from build123d import *

# Parameters (mm, degrees)
SKETCH1_R           = 5
SKETCH1_R_2         = 4.5
BOSS_EXTRUDE1_DEPTH = 15
SKETCH2_R           = 10.85
BOSS_EXTRUDE2_DEPTH = 3.5
SKETCH4_R           = 1.75
CUT_EXTRUDE1_DEPTH  = 15.5
SKETCH5_R           = 4.5
CUT_EXTRUDE2_DEPTH  = 15.5


with BuildPart() as part:
    # Sketch1 → Boss-Extrude1 (new body)
    with BuildSketch(Plane.XY):
        Circle(SKETCH1_R)
        Circle(SKETCH1_R_2, mode=Mode.SUBTRACT)
    extrude(amount=BOSS_EXTRUDE1_DEPTH)

    # Sketch2 → Boss-Extrude2 (add)
    with BuildSketch(Plane.XY.offset(4.5)):
        Circle(SKETCH2_R)
    extrude(amount=-BOSS_EXTRUDE2_DEPTH)

    # Sketch4 → Cut-Extrude1 (cut)
    with BuildSketch(Plane.XY.offset(4.5)):
        with Locations((0, 7.6)):
            Circle(SKETCH4_R)
        with Locations((7.6, 0)):
            Circle(SKETCH4_R)
        with Locations((0, -7.6)):
            Circle(SKETCH4_R)
        with Locations((-7.6, 0)):
            Circle(SKETCH4_R)
    extrude(amount=-CUT_EXTRUDE1_DEPTH, mode=Mode.SUBTRACT)

    # Sketch5 → Cut-Extrude2 (cut)
    with BuildSketch(Plane(origin=(0, 0, 1), x_dir=(-1, 0, 0), z_dir=(0, 0, -1))):
        with Locations(Location((0, 0, 0), (0, 0, 180))):
            Circle(SKETCH5_R)
    extrude(amount=-CUT_EXTRUDE2_DEPTH, mode=Mode.SUBTRACT)


solid = part.part
The model under review builds one solid part; all positions refer to its coordinate system, in mm. A direction names the side the tool comes from. Give positions to 0.01 mm unless a question says otherwise; leave off trailing zeros. Order: outer loops, then holes, each group sorted by start corner. A loop starts at its lowest first (then second) coordinate and runs counter-clockwise, first axis right, second up. Notation, with made-up numbers: M -40,58.25 L 8,58.25 A11 ccw 8,69.25 Z; hole C 2.25,12.5 d7. An arc over 180 degrees is marked long. One line per question, with ' | ' between items. Start each with the question number.
1) Wall thickness on L1, parallel to X at y = 0.25, z = 9.5; L2, parallel to X at y = -1.5, z = 4.25; L3, parallel to Y at x = 0, z = 12: over which ranges is each line inside the solid? List them lowest first. Write a range as from..to.
2) Clearance check with flat-ended pins moving along their axes: P1, Ø2, axis at x = -7.6, y = 0, coming from the -Z side; P2, Ø4, axis at x = 7.6, y = 0, coming from the +Z side; P3, Ø2, axis at y = -3, z = 12, coming from the +X side; P4, Ø4, axis at y = -5, z = 2, coming from the -X side. State where each tip first meets the part, or that it passes through.
3) Consider section C-C, the plane y = 3. Give the boundary of the cut face in (x, z), then the cut area to 3 significant figures.
4) Consider section B-B, the plane x = 8.5. Give the boundary of the cut face in (y, z).
5) Consider section D-D, the plane z = 14. Give the boundary of the cut face in (x, y).
6) Consider section A-A, the plane y = 0. Give the boundary of the cut face in (x, z).
7) Mouldability with a two-part tool opening along X and no side actions: class faces 4 (the face through (5, -2, 4.5)), 5 (the face through (-0.38, 5.89, 2.77)), 6 (the face through (-1.08, -4.88, 0.49)) as pulls with the +X half, pulls with the -X half, needs draft (parallel to the pull), parting line crosses it, or undercut.
8) For faces 1 (the face through (-8, 7.33, 2.77)), 2 (the face through (-1.08, -4.88, 9.68)), 3 (the face through (5, -2, 1)), list the 3-axis set-ups (+Z, -Z, +X, -X, +Y, -Y) from which the entire face can be reached by the end or side of a thin tool; tool diameter is ignored.
Found:
1) L1: x = -4.99..-4.49, 4.49..4.99 | L2: x = -10.75..-8.5, -6.7..-4.24, 4.24..6.7, 8.5..10.75 | L3: y = -5..-4.5, 4.5..5
2) P1: passes through | P2: stops at z = 4.5 | P3: stops at x = 4.58 | P4: stops at x = -10.43
3) outline: M -10.43,1 L -4,1 L -4,0 L -3.35,0 L -3.35,15 L -4,15 L -4,4.5 L -10.43,4.5 Z; M 3.35,0 L 4,0 L 4,1 L 10.43,1 L 10.43,4.5 L 4,4.5 L 4,15 L 3.35,15 Z | area: 64.4 mm²
4) outline: M -6.74,1 L -1.5,1 L -1.5,4.5 L -6.74,4.5 Z; M 1.5,1 L 6.74,1 L 6.74,4.5 L 1.5,4.5 Z
5) outline: C 0,0 d10; hole C 0,0 d9
6) outline: M -10.85,1 L -9.35,1 L -9.35,4.5 L -10.85,4.5 Z; M -5.85,1 L -5,1 L -5,0 L -4.5,0 L -4.5,15 L -5,15 L -5,4.5 L -5.85,4.5 Z; M 4.5,0 L 5,0 L 5,1 L 5.85,1 L 5.85,4.5 L 5,4.5 L 5,15 L 4.5,15 Z; M 9.35,1 L 10.85,1 L 10.85,4.5 L 9.35,4.5 Z
7) face 4: needs draft | face 5: undercut | face 6: parting line crosses it
8) face 1: +Z, -Z | face 2: +Z | face 3: -Z
